```python
from build123d import *

# Parameters (mm, degrees)
SKETCH2_W           = 60
SKETCH2_H           = 10
BOSS_EXTRUDE1_DEPTH = 70
SKETCH3_R           = 140
CUT_EXTRUDE1_DEPTH  = 70
BOSS_EXTRUDE2_DEPTH = 70
CUT_EXTRUDE2_REACH  = 97.669
SKETCH6_R           = 1.75
SKETCH8_R           = 3
CUT_EXTRUDE3_DEPTH  = 3


with BuildPart() as part:
    # Sketch2 → Boss-Extrude1 (new body)
    with BuildSketch(Plane(origin=(0, 0, 0), x_dir=(0, 0, -1), z_dir=(1, 0, 0))):
        with Locations((30, 5)):
            Rectangle(SKETCH2_W, SKETCH2_H)
    extrude(amount=BOSS_EXTRUDE1_DEPTH)

    # Sketch3 → Cut-Extrude1 (cut)
    with BuildSketch(Plane(origin=(70, 0, 0), x_dir=(0, 0, -1), z_dir=(1, 0, 0))):
        with Locations((73, 143.23)):
            Circle(SKETCH3_R)
    extrude(amount=-CUT_EXTRUDE1_DEPTH, mode=Mode.SUBTRACT)

    # Sketch5 → Boss-Extrude2 (add)
    with BuildSketch(Plane(origin=(70, 0, 0), x_dir=(0, 0, -1), z_dir=(1, 0, 0))):
        Polygon((60, 0), (60, 3.834878134), (64.44091692, 0), align=None)
    extrude(amount=-BOSS_EXTRUDE2_DEPTH)

    # Sketch6 → Cut-Extrude2 (cut, up to next)
    with BuildSketch(Plane(origin=(0, 10, 0), x_dir=(1, 0, 0), z_dir=(0, 1, 0)), mode=Mode.PRIVATE) as cut_extrude2_sk1:
        with Locations(Location((60, 19.991081158, 0), (0, 0, 270))):
            Circle(SKETCH6_R)
    cut_extrude2_tool1 = extrude(cut_extrude2_sk1.sketch, amount=-CUT_EXTRUDE2_REACH, mode=Mode.PRIVATE) & part.part
    # Sketch6 → Cut-Extrude2 (cut, up to next)
    with BuildSketch(Plane(origin=(0, 10, 0), x_dir=(1, 0, 0), z_dir=(0, 1, 0)), mode=Mode.PRIVATE) as cut_extrude2_sk2:
        with Locations(Location((50, 19.991081158, 0), (0, 0, 270))):
            Circle(SKETCH6_R)
    cut_extrude2_tool2 = extrude(cut_extrude2_sk2.sketch, amount=-CUT_EXTRUDE2_REACH, mode=Mode.PRIVATE) & part.part
    # Sketch6 → Cut-Extrude2 (cut, up to next)
    with BuildSketch(Plane(origin=(0, 10, 0), x_dir=(1, 0, 0), z_dir=(0, 1, 0)), mode=Mode.PRIVATE) as cut_extrude2_sk3:
        with Locations(Location((40, 19.991081158, 0), (0, 0, 270))):
            Circle(SKETCH6_R)
    cut_extrude2_tool3 = extrude(cut_extrude2_sk3.sketch, amount=-CUT_EXTRUDE2_REACH, mode=Mode.PRIVATE) & part.part
    # Sketch6 → Cut-Extrude2 (cut, up to next)
    with BuildSketch(Plane(origin=(0, 10, 0), x_dir=(1, 0, 0), z_dir=(0, 1, 0)), mode=Mode.PRIVATE) as cut_extrude2_sk4:
        with Locations(Location((30, 19.991081158, 0), (0, 0, 270))):
            Circle(SKETCH6_R)
    cut_extrude2_tool4 = extrude(cut_extrude2_sk4.sketch, amount=-CUT_EXTRUDE2_REACH, mode=Mode.PRIVATE) & part.part
    # Sketch6 → Cut-Extrude2 (cut, up to next)
    with BuildSketch(Plane(origin=(0, 10, 0), x_dir=(1, 0, 0), z_dir=(0, 1, 0)), mode=Mode.PRIVATE) as cut_extrude2_sk5:
        with Locations(Location((20, 19.991081158, 0), (0, 0, 270))):
            Circle(SKETCH6_R)
    cut_extrude2_tool5 = extrude(cut_extrude2_sk5.sketch, amount=-CUT_EXTRUDE2_REACH, mode=Mode.PRIVATE) & part.part
    # Sketch6 → Cut-Extrude2 (cut, up to next)
    with BuildSketch(Plane(origin=(0, 10, 0), x_dir=(1, 0, 0), z_dir=(0, 1, 0)), mode=Mode.PRIVATE) as cut_extrude2_sk6:
        with Locations(Location((10, 19.991081158, 0), (0, 0, 270))):
            Circle(SKETCH6_R)
    cut_extrude2_tool6 = extrude(cut_extrude2_sk6.sketch, amount=-CUT_EXTRUDE2_REACH, mode=Mode.PRIVATE) & part.part
    # Sketch6 → Cut-Extrude2 (cut, up to next)
    with BuildSketch(Plane(origin=(0, 10, 0), x_dir=(1, 0, 0), z_dir=(0, 1, 0)), mode=Mode.PRIVATE) as cut_extrude2_sk7:
        with Locations(Location((10, 9.991081158, 0), (0, 0, 270))):
            Circle(SKETCH6_R)
    cut_extrude2_tool7 = extrude(cut_extrude2_sk7.sketch, amount=-CUT_EXTRUDE2_REACH, mode=Mode.PRIVATE) & part.part
    # Sketch6 → Cut-Extrude2 (cut, up to next)
    with BuildSketch(Plane(origin=(0, 10, 0), x_dir=(1, 0, 0), z_dir=(0, 1, 0)), mode=Mode.PRIVATE) as cut_extrude2_sk8:
        with Locations(Location((20, 9.991081158, 0), (0, 0, 270))):
            Circle(SKETCH6_R)
    cut_extrude2_tool8 = extrude(cut_extrude2_sk8.sketch, amount=-CUT_EXTRUDE2_REACH, mode=Mode.PRIVATE) & part.part
    # Sketch6 → Cut-Extrude2 (cut, up to next)
    with BuildSketch(Plane(origin=(0, 10, 0), x_dir=(1, 0, 0), z_dir=(0, 1, 0)), mode=Mode.PRIVATE) as cut_extrude2_sk9:
        with Locations(Location((30, 9.991081158, 0), (0, 0, 270))):
            Circle(SKETCH6_R)
    cut_extrude2_tool9 = extrude(cut_extrude2_sk9.sketch, amount=-CUT_EXTRUDE2_REACH, mode=Mode.PRIVATE) & part.part
    # Sketch6 → Cut-Extrude2 (cut, up to next)
    with BuildSketch(Plane(origin=(0, 10, 0), x_dir=(1, 0, 0), z_dir=(0, 1, 0)), mode=Mode.PRIVATE) as cut_extrude2_sk10:
        with Locations(Location((40, 9.991081158, 0), (0, 0, 270))):
            Circle(SKETCH6_R)
    cut_extrude2_tool10 = extrude(cut_extrude2_sk10.sketch, amount=-CUT_EXTRUDE2_REACH, mode=Mode.PRIVATE) & part.part
    # Sketch6 → Cut-Extrude2 (cut, up to next)
    with BuildSketch(Plane(origin=(0, 10, 0), x_dir=(1, 0, 0), z_dir=(0, 1, 0)), mode=Mode.PRIVATE) as cut_extrude2_sk11:
        with Locations(Location((50, 9.991081158, 0), (0, 0, 270))):
            Circle(SKETCH6_R)
    cut_extrude2_tool11 = extrude(cut_extrude2_sk11.sketch, amount=-CUT_EXTRUDE2_REACH, mode=Mode.PRIVATE) & part.part
    # Sketch6 → Cut-Extrude2 (cut, up to next)
    with BuildSketch(Plane(origin=(0, 10, 0), x_dir=(1, 0, 0), z_dir=(0, 1, 0)), mode=Mode.PRIVATE) as cut_extrude2_sk12:
        with Locations(Location((60, 9.991081158, 0), (0, 0, 270))):
            Circle(SKETCH6_R)
    cut_extrude2_tool12 = extrude(cut_extrude2_sk12.sketch, amount=-CUT_EXTRUDE2_REACH, mode=Mode.PRIVATE) & part.part
    add(cut_extrude2_tool1.solids().sort_by_distance((60, 10, -19.991081))[0], mode=Mode.SUBTRACT)
    add(cut_extrude2_tool2.solids().sort_by_distance((50, 10, -19.991081))[0], mode=Mode.SUBTRACT)
    add(cut_extrude2_tool3.solids().sort_by_distance((40, 10, -19.991081))[0], mode=Mode.SUBTRACT)
    add(cut_extrude2_tool4.solids().sort_by_distance((30, 10, -19.991081))[0], mode=Mode.SUBTRACT)
    add(cut_extrude2_tool5.solids().sort_by_distance((20, 10, -19.991081))[0], mode=Mode.SUBTRACT)
    add(cut_extrude2_tool6.solids().sort_by_distance((10, 10, -19.991081))[0], mode=Mode.SUBTRACT)
    add(cut_extrude2_tool7.solids().sort_by_distance((10, 10, -9.991081))[0], mode=Mode.SUBTRACT)
    add(cut_extrude2_tool8.solids().sort_by_distance((20, 10, -9.991081))[0], mode=Mode.SUBTRACT)
    add(cut_extrude2_tool9.solids().sort_by_distance((30, 10, -9.991081))[0], mode=Mode.SUBTRACT)
    add(cut_extrude2_tool10.solids().sort_by_distance((40, 10, -9.991081))[0], mode=Mode.SUBTRACT)
    add(cut_extrude2_tool11.solids().sort_by_distance((50, 10, -9.991081))[0], mode=Mode.SUBTRACT)
    add(cut_extrude2_tool12.solids().sort_by_distance((60, 10, -9.991081))[0], mode=Mode.SUBTRACT)

    # Sketch8 → Cut-Extrude3 (cut)
    with BuildSketch(Plane.XZ):
        with Locations(Location((10, -9.991081158, 0), (0, 0, 270))):
            Circle(SKETCH8_R)
        with Locations(Location((20, -9.991081158, 0), (0, 0, 270))):
            Circle(SKETCH8_R)
        with Locations(Location((30, -9.991081158, 0), (0, 0, 270))):
            Circle(SKETCH8_R)
        with Locations(Location((40, -9.991081158, 0), (0, 0, 270))):
            Circle(SKETCH8_R)
        with Locations(Location((50, -9.991081158, 0), (0, 0, 270))):
            Circle(SKETCH8_R)
        with Locations(Location((60, -9.991081158, 0), (0, 0, 270))):
            Circle(SKETCH8_R)
        with Locations(Location((20, -19.991081158, 0), (0, 0, 270))):
            Circle(SKETCH8_R)
        with Locations(Location((30, -19.991081158, 0), (0, 0, 270))):
            Circle(SKETCH8_R)
        with Locations(Location((40, -19.991081158, 0), (0, 0, 270))):
            Circle(SKETCH8_R)
        with Locations(Location((50, -19.991081158, 0), (0, 0, 270))):
            Circle(SKETCH8_R)
        with Locations(Location((60, -19.991081158, 0), (0, 0, 270))):
            Circle(SKETCH8_R)
        with Locations(Location((10, -19.991081158, 0), (0, 0, 270))):
            Circle(SKETCH8_R)
    extrude(amount=-CUT_EXTRUDE3_DEPTH, mode=Mode.SUBTRACT)


solid = part.part
```
Work out the finished part from the listing and answer in its coordinate system (mm). A direction names the side the tool comes from. Give positions to 0.01 mm unless a question says otherwise; leave off trailing zeros. Write each loop counter-clockwise with the first axis right and the second up, starting at its lowest first coordinate (ties: lowest second). Pieces come first, ordered by that corner, then holes. Notation, with made-up numbers: (46, -29) -> (57, -29) arc R19 ccw to (57, -13) -> close; hole circle Ø5 at (30, 50). An arc over 180 degrees is marked (long way). Write each question's results on one line, items separated by ' | '.
1. Straight lines are drawn through the part: L1, parallel to Y at x = 21.5, z = -21; L2, parallel to Z at x = 29.5, y = 2.75; L3, parallel to Y at x = 55, z = -39. For each, find the intervals that lie inside material, in ascending order.
Data:
L1: 3 to 10 | L2: -61.26 to -22.95, -17.03 to -12.95, -7.03 to 0 | L3: 0 to 7.42
2. Each of these flat-tipped pins is pushed along its axis until it touches: pin 1 Ø6 at (x, y) = (11.5, 2.5) entering from -Z; pin 2 Ø5.5 at (x, z) = (30, -19.99) entering from -Y; pin 3 Ø3 at (x, z) = (60, -19.99) entering from -Y; pin 4 Ø1 at (x, z) = (60.5, -53.5) entering from +Y. Where does it stop, or does it pass through?
Data:
pin 1: z = -64.44 | pin 2: y = 3 | pin 3: through | pin 4: y = 4.67
3. Find section C-C on x = 15.5. Determine the outline of the cut face in (y, z), and give its area (3 significant figures).
Data:
outline: (0, -64.44) -> (3.83, -60) arc R140 cw to (10, -29.99) -> (10, 0) -> (0, 0) -> close | area: 499 mm^2
4. Find section B-B on y = 1.5. Give the number of separate pieces and of enclosed holes in the cut face, and give its area (3 significant figures).
Data:
separate pieces: 1 | enclosed holes: 12 | area: 4,050 mm^2
5. A tool of negligible diameter and unlimited length cuts with its end or side. For faces 1 (the flat face through (38, 3, -20)), 2 (the cylindrical face through (11.476, 6.549, -19.05)), from which of +Z, -Z, +X, -X, +Y, -Y can it reach the whole face along a straight path? Write none if from no direction.
Data:
face 1: -Y | face 2: +Y, -Y
6. Determine the mould class of faces 3 (the flat face through (28, 3, -20)), 4 (the flat face through (35, 0, -33)) for opening direction X: +X half, -X half, draft (parallel to the pull), parting line (faces both ways), or undercut.
Data:
face 3: undercut | face 4: draft
7. Find section A-A on x = 60. Determine the outline of the cut face in (y, z), and give its area (3 significant figures).
Data:
outline: (0, -64.44) -> (3.83, -60) arc R140 cw to (10, -29.99) -> (10, -21.74) -> (3, -21.74) -> (3, -22.99) -> (0, -22.99) -> close; (0, -16.99) -> (3, -16.99) -> (3, -18.24) -> (10, -18.24) -> (10, -11.74) -> (3, -11.74) -> (3, -12.99) -> (0, -12.99) -> close; (0, -6.99) -> (3, -6.99) -> (3, -8.24) -> (10, -8.24) -> (10, 0) -> (0, 0) -> close | area: 414 mm^2
